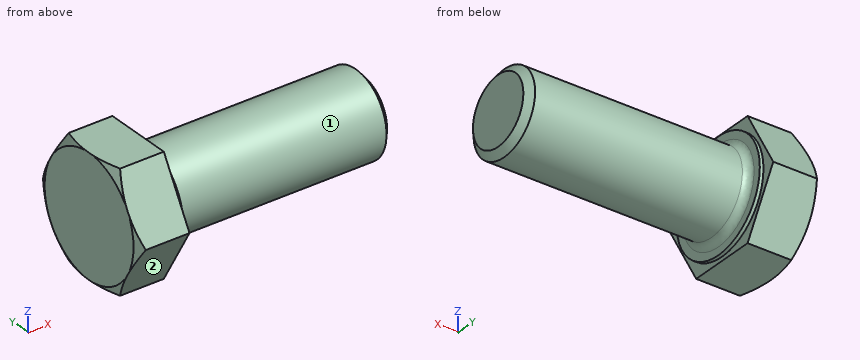
Autodesk Inventor part; units mm, degrees
ref_plane "Work Plane1" through (1.525, 0, 0) normal (0, 0, 1) x (1, 0, 0)
ref_plane "YZ Plane" through (0, 0, 0) normal (1, 0, 0) x (0, 1, 0)
ref_plane "XZ Plane" through (0, 0, 0) normal (0, 1, 0) x (-1, 0, 0)
sketch "Sketch1" plane through (0, 0, 0) normal (0, 0, 1) x (1, 0, 0)
  line L0 (0, 9.6441) -> (0, 7.1437)
  line L1 (3.175, 7.1437) -> (38.1, 7.1438)
  line L2 (38.1, 7.1438) -> (38.1, 0)
  line L3 (38.1, 0) -> (-0.6351, 0)
  line L4 (-8.3821, 0) -> (45.847, 0)
  line L5 (-0.6351, 0) -> (-0.6351, 9.6441)
  line L6 (-0.6351, 9.6441) -> (0, 9.6441)
  line L7 (3.175, 7.1437) -> (1.0582, 7.1437)
  line L8 (1.0582, 7.1437) -> (0, 7.1437)
  line L9 (0, -1.9288) -> (0, 11.5729)
  dimension "d0" = 38.1
  dimension "d1" = 34.925
  dimension "d2" = 14.2875
  dimension "d9" = 0.6351
  dimension "d10" = 19.2881
  dimension "d13" = 2.1168
  dimension "d14" = 14.2875
revolve "Body" add sketch "Sketch1" angle 360 about axis through (38.1, 0, 0) along (-1, 0, 0)
sketch "Sketch2" plane through (-0.6351, 0, 0) normal (-1, 0, 0) x (0, 0, 1)
  line L0 (0, 11.9151) -> (10.3187, 5.9575)
  line L1 (10.3187, 5.9575) -> (10.3187, -5.9575)
  line L2 (10.3187, -5.9575) -> (0, -11.9151)
  line L3 (0, -11.9151) -> (-10.3187, -5.9575)
  line L4 (-10.3187, -5.9575) -> (-10.3187, 5.9575)
  line L5 (-10.3187, 5.9575) -> (0, 11.9151)
  point P0 (0, 0)
  point P1 (0, 0)
  dimension "d11" = 20.6375
extrude "Head" add sketch "Sketch2" along normal blind 8.4931
sketch "Sketch4" plane through (0, 0, 0) normal (0, 0, 1) x (1, 0, 0)
  line L0 (-9.1282, 10.3188) -> (-9.1282, 11.9151)
  line L1 (-9.1282, 11.9151) -> (-8.2066, 11.9151)
  line L2 (-8.2066, 11.9151) -> (-9.1282, 10.3188)
  line L3 (-10.8269, 0) -> (1.0635, 0)
  line L4 (-0.6351, 11.9151) -> (-9.1282, 11.9151)
  line L5 (-9.1282, 5.9575) -> (-9.1282, 11.9151)
  dimension "d5" = 30
  dimension "d19" = 20.6375
revolve "Chamfer1" cut sketch "Sketch4" angle 360 about axis through (-10, 0, 0) along (1, 0, 0)
thread "Thread"
chamfer "Chamfer2" distance 1.2985 distance2 1.0584 1 edges at (38.1, -7.1437, 0) measured on face at (38.1, -1.2527, -0.5699)
ref_plane "Work Plane1" through (1.525, 0, 0) normal (0, 0, 1) x (1, 0, 0)
fillet "Fillet2" radius 1.143 1 edges at (0, -7.1437, 0)
equation "\"d0\" = NLG"
equation "\"d1\" = GEL"
equation "\"d2\" = GD"
equation "\"d10\" = SD2"
equation "\"d14\" = BDM"
equation "\"d11\" = SW"
equation "\"d3\" = KOH - SD"
equation "\"d5\" = ANG1"
equation "\"d19\" = SW0"
equation "\"d63\" = R"
equation "\"d15\" = GEL"
equation "\"d6\" = -0.5 * SPD + 0.5 * GD"
equation "\"NLG\" = 38.1"
equation "\"GD\" = NND"
equation "\"BDM\" = 14.2875"
equation "\"KOH\" = 9.12813"
equation "\"GEL\" = 34.925"
equation "\"SW\" = 20.6375"
equation "\"SW0\" = SW"
equation "\"SPD\" = 11.69055"
equation "\"SD2\" = 19.28813"
equation "\"SD\" = 0.635"
equation "\"ANG1\" = 30deg"
equation "\"GAL\" = 2.11667"
equation "\"GUL\" = 1.05833"
equation "\"R\" = 1.143"
equation "\"THREADDIA\" = 14.2875"
equation "\"TOA\" = 30deg"
equation "\"RR\" = 0.762"
equation "\"NND\" = 14.2875"
equation "\"E0\" = 1.155 * SW"
equation "\"SLG\" = 0"
equation "\"GD1\" = 11.69055"
properties part number "ANSI B18.2.1 - 9/16-12 UNC - 1.5, HCSI" material "Steel, Mild"
Source: CAD feature listing. Evaluate the final solid. Frame: model axes, mm. Face numbers are marked on the shaded views. A direction names the side the tool comes from. Round coordinates to 2 decimals unless told otherwise and drop trailing zeros. Loops run counter-clockwise (first coordinate to the right, second up) from the corner with the lowest first, then second, coordinate; pieces in that order, holes last. Notation, with made-up numbers: M -1.5,77 L 16.5,77 A34 cw 16.5,114 Z; hole C 26.25,-35 d8. An arc over 180 degrees is marked long. Put each result on its own line as item: value.
(1) Section B-B, the plane x = 20.5. Return loops of the section in (y, z).
Solutions:
outline: C 0,0 d14.29
(2) Ray query, line 1 (X direction, y = 6, z = -6.25); line 2 (X direction, y = 9, z = 3.75); line 3 (Y direction, x = -6.5, z = 5.25). Return the intervals inside material, ascending. Write a range as [from, to].
Solutions:
line 1: [-9.13, 0]
line 2: [-9.13, -0.64]
line 3: [-8.88, 8.88]
(3) First-contact query: pin 1 (5 mm diameter, centred on x = 21, y = -8.5, fed in from +Z); pin 2 (8 mm diameter, centred on x = 20.5, z = 6.5, fed in from -Y); pin 3 (3 mm diameter, centred on x = 19, z = -1.5, fed in from -Y). Flat tips, straight axial feed; report the tip coordinate or a pass-through.
Solutions:
pin 1: z = 3.88
pin 2: y = -6.69
pin 3: y = -7.14
(4) Access query for the marked faces 1 and 2. Directions: +Z, -Z, +X, -X, +Y, -Y. A direction counts if a zero-diameter tool reaches every point of the face in a straight line with its end or side. Return the directions, or none.
Solutions:
face 1: +X
face 2: -Z, +X, -X, -Y
(5) Section A-A, the plane x = -4. Return loops of the section in (y, z), and give its area (3 significant figures).
Solutions:
outline: M -11.92,0 L -5.96,-10.32 L 5.96,-10.32 L 11.92,0 L 5.96,10.32 L -5.96,10.32 Z
area: 369 mm²
